```python
from build123d import *

# Parameters (mm, degrees)
ENL_V_MAT_EXTRU_1_REACH      = 24
ESQUISSE2_R                  = 1.75
ENL_V_MAT_EXTRU_2_DEPTH      = 10
R_P_TITION_CIRCULAIRE1_COUNT = 24


with BuildPart() as part:
    # Esquisse1 → Révolution1 (revolve)
    with BuildSketch(Plane.XY):
        Polygon((0, 2.25), (0, 5.05), (13, 5.05), (13, 8), (16, 8), (16, 15), (22, 15), (22, 2.6), (6, 2.6), (6, 1.2), (3, 1.2), (3, 2.25), align=None)
    revolve(axis=Axis((0, 0, 0), (1, 0, 0)))

    # Esquisse2 → Enlèv. mat.-Extru.1 (cut, up to next)
    with BuildSketch(Plane(origin=(22, 0, 0), x_dir=(0, 0, -1), z_dir=(1, 0, 0)), mode=Mode.PRIVATE) as enl_v_mat_extru_1_sk1:
        with Locations((0, 11)):
            Circle(ESQUISSE2_R)
    enl_v_mat_extru_1_tool1 = extrude(enl_v_mat_extru_1_sk1.sketch, amount=-ENL_V_MAT_EXTRU_1_REACH, mode=Mode.PRIVATE) & part.part
    add(enl_v_mat_extru_1_tool1.solids().sort_by_distance((22, 11, 0))[0], mode=Mode.SUBTRACT)
    # Esquisse2 → Enlèv. mat.-Extru.1 (cut, up to next)
    with BuildSketch(Plane(origin=(22, 0, 0), x_dir=(0, 0, -1), z_dir=(1, 0, 0)), mode=Mode.PRIVATE) as enl_v_mat_extru_1_sk2:
        with Locations((11, 0)):
            Circle(ESQUISSE2_R)
    enl_v_mat_extru_1_tool2 = extrude(enl_v_mat_extru_1_sk2.sketch, amount=-ENL_V_MAT_EXTRU_1_REACH, mode=Mode.PRIVATE) & part.part
    add(enl_v_mat_extru_1_tool2.solids().sort_by_distance((22, 0, -11))[0], mode=Mode.SUBTRACT)
    # Esquisse2 → Enlèv. mat.-Extru.1 (cut, up to next)
    with BuildSketch(Plane(origin=(22, 0, 0), x_dir=(0, 0, -1), z_dir=(1, 0, 0)), mode=Mode.PRIVATE) as enl_v_mat_extru_1_sk3:
        with Locations((0, -11)):
            Circle(ESQUISSE2_R)
    enl_v_mat_extru_1_tool3 = extrude(enl_v_mat_extru_1_sk3.sketch, amount=-ENL_V_MAT_EXTRU_1_REACH, mode=Mode.PRIVATE) & part.part
    add(enl_v_mat_extru_1_tool3.solids().sort_by_distance((22, -11, 0))[0], mode=Mode.SUBTRACT)
    # Esquisse2 → Enlèv. mat.-Extru.1 (cut, up to next)
    with BuildSketch(Plane(origin=(22, 0, 0), x_dir=(0, 0, -1), z_dir=(1, 0, 0)), mode=Mode.PRIVATE) as enl_v_mat_extru_1_sk4:
        with Locations((-11, 0)):
            Circle(ESQUISSE2_R)
    enl_v_mat_extru_1_tool4 = extrude(enl_v_mat_extru_1_sk4.sketch, amount=-ENL_V_MAT_EXTRU_1_REACH, mode=Mode.PRIVATE) & part.part
    add(enl_v_mat_extru_1_tool4.solids().sort_by_distance((22, 0, 11))[0], mode=Mode.SUBTRACT)

    # Esquisse3 → Enlèv. mat.-Extru.2 (cut)
    with BuildSketch(Plane.ZY.offset(-3)):
        Polygon((2.54609184, 0), (2.163423814, -0.382668026), (2.164412287, 0.381679553), align=None)
    enl_v_mat_extru_2 = extrude(amount=ENL_V_MAT_EXTRU_2_DEPTH, mode=Mode.SUBTRACT)

    # Répétition circulaire1: Enlèv. mat.-Extru.2 ×24 about axis
    r_p_tition_circulaire1_axis = Axis((0, 0, 0), (1, 0, 0))
    for i in range(1, R_P_TITION_CIRCULAIRE1_COUNT):
        add(enl_v_mat_extru_2.rotate(r_p_tition_circulaire1_axis, i * 360 / R_P_TITION_CIRCULAIRE1_COUNT), mode=Mode.SUBTRACT)


solid = part.part
```
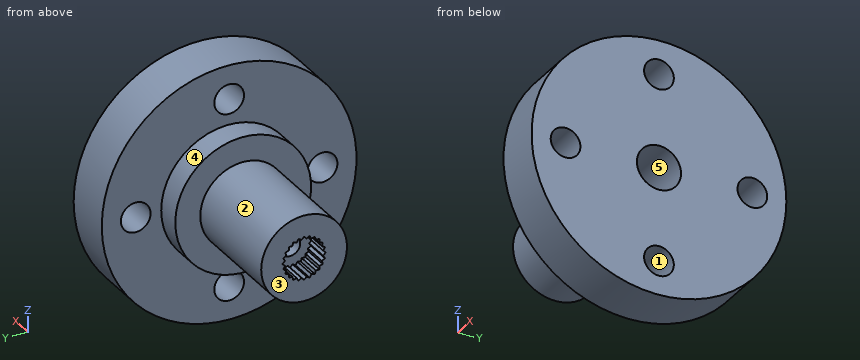
Model file for the job. Use its own axes, mm. Face numbers are marked on the shaded views. A direction names the side the tool comes from. Give positions to 0.01 mm unless a question says otherwise; leave off trailing zeros. Loops run counter-clockwise (first coordinate to the right, second up) from the corner with the lowest first, then second, coordinate; pieces in that order, holes last. Notation, with made-up numbers: (59, 13) - (112, 13) arc R25 cw to (112, 49) - close; hole circle Ø3 at (56, 10). An arc over 180 degrees is marked (long way). One line per item, written item: value. Start each with the question number.
1. Slice it at A-A (z = -11). List the corners of the cut face in (x, y).
2. Which spindle directions (+Z, -Z, +X, -X, +Y, -Y) get a long thin tool onto all of the face, cutting with end or side? Do the marked faces 1 and 2. Say none if no direction does.
3. Pull direction Y, two halves, no side cores. Call the marked faces 3, 4 and 5: pulls with the +Y half, pulls with the -Y half, needs draft (parallel to the pull), parting line crosses it, or undercut.
4. Pin check, flat tips, straight feed: pin 1 (5.5 mm diameter, centred on y = -1, z = -0.5, fed in from -X); pin 2 (3 mm diameter, centred on y = 0, z = 0, fed in from -X); pin 3 (3 mm diameter, centred on y = 11, z = 0, fed in from +X); pin 4 (0.5 mm diameter, centred on x = 1.5, y = -1.5, fed in from +Z). Stop position of each tip, or through.
5. Slice it at D-D (y = -6.5). List the corners of the cut face in (x, z).
6. Slice it at C-C (x = 18.25). List the corners of the cut face in (y, z), plus the area to 3 significant figures.
7. Probe L1, parallel to Z at x = 3.7, y = 0; L2, parallel to X at y = 3.25, z = 11.5; L3, parallel to Z at x = 10, y = 1. List the from-to ranges inside material, lowest first. Write a range as from..to.
Solution:
1. outline: (16, -10.2) - (22, -10.2) - (22, -1.75) - (16, -1.75) - close; (16, 1.75) - (22, 1.75) - (22, 10.2) - (16, 10.2) - close
2. face 1: +X, -X
2. face 2: -X
3. face 3: needs draft
3. face 4: parting line crosses it
3. face 5: undercut
4. pin 1: stops at x = 0
4. pin 2: stops at x = 3
4. pin 3: passes through
4. pin 4: stops at z = 4.89
5. outline: (13, -4.66) - (16, -4.66) - (16, -13.52) - (22, -13.52) - (22, 13.52) - (16, 13.52) - (16, 4.66) - (13, 4.66) - close
6. outline: circle Ø30 at (0, 0); hole circle Ø3.5 at (-11, 0); hole circle Ø5.2 at (0, 0); hole circle Ø3.5 at (0, -11); hole circle Ø3.5 at (0, 11); hole circle Ø3.5 at (11, 0)
6. area: 647 mm^2
7. L1: z = -5.05..-1.2, 1.2..5.05
7. L2: x = 16..22
7. L3: z = -4.95..-2.4, 2.4..4.95
